Read the model definition and answer for the solid it produces. Units are mm, in the model's axes. A direction names the side the tool comes from. Coordinates: 2 decimals unless noted, no trailing zeros. Order: outer loops, then holes, each group sorted by start corner. A loop starts at its lowest first (then second) coordinate and runs counter-clockwise, first axis right, second up.
Autodesk Inventor part; units mm, degrees
ref_plane "Work Plane1" through (0, 0, 0) normal (0, -1, 0) x (1, 0, 0)
ref_plane "Work Plane2" through (0, 0, 11.5) normal (0, 0, 1) x (1, 0, 0)
ref_plane "XZ Plane" through (0, 0, 0) normal (0, 1, 0) x (-1, 0, 0)
sketch "Sketch1" plane through (0, 0, 0) normal (0, 1, 0) x (-1, 0, 0)
  line L0 (20, 0) -> (20, -8) construction
  line L1 (20, -8) -> (20, 8)
  line L2 (20, 8) -> (0, 8)
  line L3 (20, -8) -> (0, -8)
  line L4 (0, -8) -> (-2.0965, -19.8898)
  line L5 (0, 8) -> (-2.0965, 19.8898)
  arc A0 (-2.0965, 19.8898) -> (-2.0965, -19.8898) centre (0, 0) ccw construction
  arc A1 (18.3303, -8) -> (18.3303, 8) centre (0, 0) ccw construction
  arc A2 (-2.0965, 19.8898) -> (-2.0965, -19.8898) centre (0, 0) ccw
  arc A3 (18.3303, -8) -> (18.3303, 8) centre (0, 0) ccw
  circle A4 centre (0, 0) radius 20 construction
  circle A5 centre (13, 0) radius 4
  circle A6 centre (0, 0) radius 4
  circle A7 centre (0, 0) radius 6.5
  dimension "d1" = 8
  dimension "d2" = 16
  dimension "d3" = 20
  dimension "d4" = 20
  dimension "d5" = 100
  dimension "d6" = 100
  dimension "d7" = 40
  dimension "d8" = 20
  dimension "d10" = 8
  dimension "d14" = 8
  dimension "d15" = 13
  dimension "d16" = 13
  dimension "d21" = 7
extrude "Extrusion4" add sketch "Sketch1" along normal blind 7 contours A3 L3 L4 A2 L5 L2
extrude "Extrusion5" add sketch "Sketch1" along normal blind 7.8 contours A7
fillet "Fillet1" radius 4 1 edges at (-18.3303, 3.5, 8)
fillet "Fillet2" radius 4 1 edges at (-18.3303, 3.5, -8)
fillet "Fillet3" radius 4 2 edges at (0, 3.5, -8) (0, 3.5, 8)
fillet "Fillet4" radius 1 2 edges at (2.0965, 3.5, 19.8898) (2.0965, 3.5, -19.8898)
ref_plane "Work Plane1" through (0, 0, 0) normal (0, -1, 0) x (1, 0, 0)
sketch "Sketch3" plane through (-15.4919, 0, 8) normal (0, 0, 1) x (1, 0, 0)
  line L0 (6.4919, 0) -> (-1.5081, 0)
  line L1 (0, 7) -> (12.1355, 7)
  line L2 (-3.873, 7) -> (0, 7)
  line L3 (0, 0) -> (-3.873, 0)
  line L4 (-1.5081, 7) -> (6.4919, 7)
  line L5 (6.4919, 0) -> (-1.5081, 0)
  line L6 (19.4919, 0) -> (11.4919, 0)
  line L7 (6.4919, 0) -> (-1.5081, 0)
  line L8 (18.5607, 0) -> (17.4225, 0)
  line L9 (18.5607, 0) -> (18.5607, 0)
  line L10 (17.4225, 0) -> (18.5607, 0)
  line L11 (16.0748, 0) -> (17.4225, 0)
  line L12 (12.1355, 0) -> (16.0748, 0)
  line L13 (0, 0) -> (12.1355, 0)
  line L14 (-3.873, 0) -> (0, 0)
  line L15 (-3.873, 0) -> (-3.873, 0)
  line L16 (0, 0) -> (-3.873, 0)
  line L17 (12.1355, 0) -> (0, 0)
  line L18 (16.0748, 0) -> (12.1355, 0)
  line L19 (17.4225, 0) -> (16.0748, 0)
  circle A0 centre (1.1355, 3.4977) radius 1.25
  line L20 (12.1355, 7) -> (12.1355, 0)
  point P0 (15.4919, 0)
  dimension "d33" = 2.5
  dimension "d34" = 11
  dimension "d35" = 3.4977
extrude "Extrusion6" cut sketch "Sketch3" against normal through all
ref_plane "Work Plane2" through (0, 0, 11.5) normal (0, 0, 1) x (1, 0, 0)
sketch "Sketch5" plane through (0, 0, 11.5) normal (0, 0, 1) x (1, 0, 0)
  line L0 (0.5828, 0) -> (0.5828, 7)
  line L1 (0.5828, 0) -> (1.9305, 0) construction
  line L2 (0.5828, 0) -> (-4.4172, 0) construction
  line L3 (-4.4172, 0) -> (-4.4172, 7) construction
  line L4 (-4.4172, 7) -> (0.5828, 7) construction
  line L5 (-4.4172, 0) -> (-4.4172, 3.5) construction
  line L6 (-4.4172, 7) -> (-1.9172, 7) construction
  circle A0 centre (-1.9172, 3.5) radius 1.25
  point P0 (0, 0)
  dimension "d45" = 5
  dimension "d46" = 7
  dimension "d47" = 5
  dimension "d48" = 3.5
  dimension "d50" = 2.5
extrude "Extrusion7" cut sketch "Sketch5" against normal through all
properties part number "reverse gear crankshaft counter weight 2"
1) Straight lines are drawn through the part: line 1 (X direction, y = 6.25, z = -2.5); line 2 (X direction, y = 3.5, z = 5.5); line 3 (Z direction, x = 0, y = 2.25). For each, find the intervals that lie inside material, in ascending order.
A:
line 1: x = -19.84 to -16.12, -9.88 to -3.12, 3.12 to 19.84
line 2: x = -19.2 to -15.61, -13.11 to -3.17, -0.67 to 19.23
line 3: z = -9.82 to -4, 4 to 9.82
2) A cutting plane is placed at D-D, the plane x = 10.5. Determine the outline of the cut face in (y, z).
A:
outline: (0, -17.02) - (7, -17.02) - (7, 17.02) - (0, 17.02) - close
3) A cutting plane is placed at C-C, the plane z = -5.5. Determine the outline of the cut face in (x, y), and give its area (3 significant figures).
A:
outline: (-19.2, 0) - (19.23, 0) - (19.23, 7) - (3.46, 7) - (3.46, 7.8) - (-3.46, 7.8) - (-3.46, 7) - (-19.2, 7) - close; hole circle Ø2.5 at (-14.36, 3.5); hole circle Ø2.5 at (-1.92, 3.5)
area: 265 mm2
4) Determine the mould class of faces 4 (the cylindrical face through (-0.37, 3.55, -9.34)), 5 (the flat face through (-3, 7.8, 3)), 6 (the cylindrical face through (-15.605, 3.553, 6.103)), 7 (the cylindrical face through (20, 3, 0)) for opening direction X: pulls with the +X half, pulls with the -X half, needs draft (parallel to the pull), parting line crosses it, or undercut.
A:
face 4: pulls with the -X half
face 5: needs draft
face 6: undercut
face 7: pulls with the +X half
5) Which of the six approach directions +Z, -Z, +X, -X, +Y, -Y give full straight-line access (tool end or side, diameter ignored) to faces 1 (the cylindrical face through (-20, 3, 0)), 2 (the flat face through (-10, 3, -8)), 3 (the flat face through (-10, 3, 8))?
A:
face 1: -X, +Y, -Y
face 2: -Z, -X, +Y, -Y
face 3: +Z, -X, +Y, -Y
6) A cutting plane is placed at B-B, the plane x = 0. Determine the outline of the cut face in (y, z), and give its area (3 significant figures).
A:
outline: (0, -9.82) - (7, -9.82) - (7, -6.5) - (7.8, -6.5) - (7.8, -4) - (0, -4) - close; (0, 4) - (7.8, 4) - (7.8, 6.5) - (7, 6.5) - (7, 9.82) - (0, 9.82) - close
area: 85.5 mm2
7) A cutting plane is placed at A-A, the plane z = 0. Determine the outline of the cut face in (x, y), and give its area (3 significant figures).
A:
outline: (-20, 0) - (-17, 0) - (-17, 7) - (-20, 7) - close; (-9, 0) - (-4, 0) - (-4, 7.8) - (-6.5, 7.8) - (-6.5, 7) - (-9, 7) - close; (4, 0) - (20, 0) - (20, 7) - (6.5, 7) - (6.5, 7.8) - (4, 7.8) - close
area: 172 mm2
8) Flat-ended cylindrical pins translate along their axes: pin 1 Ø3.5 at (x, y) = (-11.5, 4) entering from +Z; pin 2 Ø10.5 at (x, z) = (-13, 0) entering from +Y; pin 3 Ø3.5 at (x, y) = (-12, 4.5) entering from -Z; pin 4 Ø2 at (x, y) = (-14.36, 3.5) entering from +Z (1 decimal). Find the tip coordinate at first contact, or state that the pin passes through.
A:
pin 1: stops at z = 8
pin 2: stops at y = 7
pin 3: stops at z = -8
pin 4: passes through
